Can you work these out from the model? Positions are in its coordinate system, mm. A direction names the side the tool comes from. Round coordinates to 2 decimals unless told otherwise and drop trailing zeros. Loops run counter-clockwise (first coordinate to the right, second up) from the corner with the lowest first, then second, coordinate; pieces in that order, holes last. Notation, with made-up numbers: (84, 24) -> (113, 24) arc R19 cw to (113, 44) -> close; hole circle Ø1 at (-15.5, 35). An arc over 180 degrees is marked (long way). Write item = value, one per line.
from build123d import *

# Parameters (mm, degrees)
EXTRUDE_1_DEPTH          = 7
CUT_EXTRUDE_3_DEPTH      = 2.5
CUT_EXTRUDE_6_DEPTH      = 2.5
CUT_EXTRUDE_6_DEPTH_BACK = 2.5
SKETCH_11_R              = 3.5
EXTRUDE_4_DEPTH          = 10
EXTRUDE_START            = -10
SKETCH_13_R              = 3.5
EXTRUDE_5_DEPTH          = 10
SKETCH_12_W              = 2.5
SKETCH_12_H              = 8.803448755
SKETCH_12_W_2            = 2.746212411
SKETCH_12_H_2            = 8.519621178
CUT_EXTRUDE_10_DEPTH     = 10
CHAMFER_1_SIZE           = 0.5
CHAMFER_2_SIZE           = 0.5
FILLET_1_R               = 0.5
SKETCH_14_R              = 1.5
CUT_EXTRUDE_11_DEPTH     = 123


with BuildPart() as part:
    # Sketch 2 → Extrude 1 (new body)
    with BuildSketch(Plane(origin=(0, 0, 0), x_dir=(1, 0, 0), z_dir=(0, 1, 0))):
        with BuildLine():
            Line((-35, 0), (-25, 0))
            ThreePointArc((-25, 0), (0, 25), (25, 0))
            Line((25, 0), (35, 0))
            ThreePointArc((35, 0), (0, 35), (-35, 0))
        make_face()
    extrude(amount=EXTRUDE_1_DEPTH)

    # Sketch 3 → Cut-Extrude 3 (cut)
    with BuildSketch(Plane(origin=(0, 7, 0), x_dir=(1, 0, 0), z_dir=(0, 1, 0))):
        with BuildLine():
            Line((26.076809621, 7), (32.249030993, 7))
            ThreePointArc((32.249030993, 7), (0, 33), (-32.249030993, 7))
            Line((-32.249030993, 7), (-26.076809621, 7))
            ThreePointArc((-26.076809621, 7), (0, 27), (26.076809621, 7))
        make_face()
    extrude(amount=-CUT_EXTRUDE_3_DEPTH, mode=Mode.SUBTRACT)

    # Sketch 5 → Cut-Extrude 6 (cut, two sides: drawn at the far end of the back side and taken through both)
    with BuildSketch(Plane(origin=(0, 0, 0), x_dir=(1, 0, 0), z_dir=(0, 1, 0)).offset(-CUT_EXTRUDE_6_DEPTH_BACK)):
        with BuildLine():
            Line((26.160532749, 7), (32.316767687, 7))
            ThreePointArc((32.316767687, 7), (0, 33.319691154), (-32.316767687, 7))
            Line((-32.316767687, 7), (-26.160532749, 7))
            ThreePointArc((-26.160532749, 7), (0, 27.319691154), (26.160532749, 7))
        make_face()
    extrude(amount=CUT_EXTRUDE_6_DEPTH + CUT_EXTRUDE_6_DEPTH_BACK, mode=Mode.SUBTRACT)

    # Sketch 11 → Extrude 4 (add)
    with BuildSketch(Plane.ZY.offset(35)):
        with Locations((0, 3.5)):
            Circle(SKETCH_11_R)
    extrude(amount=-EXTRUDE_4_DEPTH)

    # Sketch 13 → Extrude 5 (add)
    with BuildSketch(Plane(origin=(35, 0, 0), x_dir=(0, 0, -1), z_dir=(1, 0, 0)).offset(EXTRUDE_START)):
        with Locations((0, 3.5)):
            Circle(SKETCH_13_R)
    extrude(amount=EXTRUDE_5_DEPTH)

    # Sketch 12 → Cut-Extrude 10 (cut)
    with BuildSketch(Plane(origin=(0, 7, 0), x_dir=(1, 0, 0), z_dir=(0, 1, 0))):
        with Locations((-33.75, -0.901724378)):
            Rectangle(SKETCH_12_W, SKETCH_12_H)
        with Locations((-28.75, -0.901724378)):
            Rectangle(SKETCH_12_W, SKETCH_12_H)
        with Locations((26.126893794, -0.759810589)):
            Rectangle(SKETCH_12_W_2, SKETCH_12_H_2)
        with Locations((31.25, -0.759810589)):
            Rectangle(SKETCH_12_W, SKETCH_12_H_2)
    extrude(amount=-CUT_EXTRUDE_10_DEPTH, mode=Mode.SUBTRACT)

    # Chamfer 1
    chamfer_1_edges = [part.edges().sort_by_distance(p)[0] for p in [
        (0, 7, -33),
        (-29.162920307, 7, -7),
        (0, 7, -27),
        (29.162920307, 7, -7),
    ]]
    chamfer(chamfer_1_edges, length=CHAMFER_1_SIZE)

    # Chamfer 2
    chamfer_2_edges = [part.edges().sort_by_distance(p)[0] for p in [
        (29.238650218, 0, -7),
        (0, 0, -27.319691154),
        (-29.238650218, 0, -7),
        (0, 0, -33.319691154),
    ]]
    chamfer(chamfer_2_edges, length=CHAMFER_2_SIZE)

    # Fillet 1
    fillet_1_edges = [part.edges().sort_by_distance(p)[0] for p in [
        (26.126893794, 0, -3.5),
        (24.753787589, 3.5, -3.5),
        (26.126893794, 7, -3.5),
        (31.25, 0, -3.5),
        (31.25, 7, -3.5),
        (-33.662280149, 0, -3.5),
        (-34.824560299, 3.5, -3.5),
        (-33.662280149, 7, -3.5),
        (-28.75, 0, -3.5),
        (-28.75, 7, -3.5),
    ]]
    fillet(fillet_1_edges, radius=FILLET_1_R)

    # Sketch 14 → Cut-Extrude 11 (cut)
    with BuildSketch(Plane(origin=(35, 0, 0), x_dir=(0, 0, -1), z_dir=(1, 0, 0))):
        with Locations((0, 3.5)):
            Circle(SKETCH_14_R)
    extrude(amount=-CUT_EXTRUDE_11_DEPTH, mode=Mode.SUBTRACT)


solid = part.part
1. For faces 4 (the conical face through (-0.643, 0.365, -33.449)), 5 (the conical face through (0.638, 6.635, -33.129)), 6 (the flat face through (31, 4, -3.5)), which set-ups out of +Z, -Z, +X, -X, +Y, -Y let a thin tool reach every point of the face, with its end or its side?
Entries:
face_4 = -Y
face_5 = +Y
face_6 = +Z, +Y, -Y
2. Suppose I cut it at A-A, the plane x = 0. List the corners of the cut face in (y, z) for me, and give its area (3 significant figures).
Entries:
outline = (0, -35) -> (7, -35) -> (7, -33.5) -> (6.5, -33) -> (4.5, -33) -> (4.5, -27) -> (6.5, -27) -> (7, -26.5) -> (7, -25) -> (0, -25) -> (0, -26.82) -> (0.5, -27.32) -> (2.5, -27.32) -> (2.5, -33.32) -> (0.5, -33.32) -> (0, -33.82) -> close
area = 39.5 mm²
3. Suppose I cut it at B-B, the plane y = 3.5. Count the separate pieces of the cut face and the enclosed holes in it, and give its area (3 significant figures).
Entries:
separate_pieces = 5
enclosed_holes = 0
area = 912 mm²
4. I'm going to push flat-ended pins straight in: pin 1 (3 mm diameter, centred on y = 5.5, z = -17, fed in from +X); pin 2 (3 mm diameter, centred on y = 4.5, z = -15, fed in from +X); pin 3 (3.5 mm diameter, centred on y = 3.5, z = 0, fed in from -X). Where does each tip first touch, or does it pass through?
Entries:
pin_1 = 31.38
pin_2 = 32.29
pin_3 = -32.5
5. We'd pull the mould along X, two halves only. Please class faces 1 (the flat face through (35, 4, -2)), 2 (the cylindrical face through (-26.3, 3.4, 3.5)), 3 (the conical face through (-0.498, 0.142, -26.957)): released by +X, released by -X, zero draft, split by the parting line, or undercut.
Entries:
face_1 = released by +X
face_2 = zero draft
face_3 = undercut
6. I need wall thicknesses on line 1 (X direction, y = 0.5, z = -9); line 2 (X direction, y = 6, z = -9); line 3 (Y direction, x = -26.3, z = 0). Which ranges of each line are inside material? Lowest first, please. Write a range as [from, to].
Entries:
line_1 = [-33.82, -31.84], [-25.57, -23.32], [23.32, 25.57], [31.84, 33.82]
line_2 = [-33.82, -31.75], [-25.46, -23.32], [23.32, 25.46], [31.75, 33.82]
line_3 = [0, 2], [5, 7]
